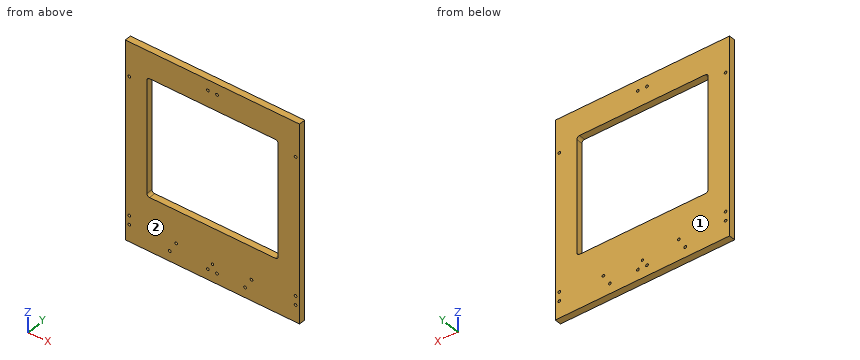
```python
from build123d import *

# Parameters (mm, degrees)
SKETCH_W        = 324
SKETCH_H        = 370
PAD_DEPTH       = 12
POCKET_DEPTH    = 12.001
SKETCH002_R     = 2.5
POCKET001_DEPTH = 12.001
SKETCH003_R     = 2.5
SKETCH003_R_2   = 2.25
POCKET002_DEPTH = 12.001


with BuildPart() as part:
    # Sketch → Pad (new body)
    with BuildSketch(Plane.XZ):
        with Locations((0, 185)):
            Rectangle(SKETCH_W, SKETCH_H)
    extrude(amount=PAD_DEPTH)

    # Sketch001 → Pocket (cut, through all)
    with BuildSketch(Plane.XZ.offset(12)):
        with BuildLine():
            ThreePointArc((-116.999969, 320), (-120.535523, 318.535545), (-122, 315))
            Line((-122, 315), (-122, 105))
            ThreePointArc((-122, 105), (-120.535523, 101.464455), (-116.999969, 100))
            Line((-116.999969, 100), (116.999969, 100))
            ThreePointArc((116.999969, 100), (120.535503, 101.464466), (121.999969, 105))
            Line((121.999969, 105), (121.999969, 315))
            ThreePointArc((121.999969, 315), (120.535503, 318.535534), (116.999969, 320))
            Line((-116.999969, 320), (116.999969, 320))
        make_face()
    extrude(amount=-POCKET_DEPTH, mode=Mode.SUBTRACT)

    # Sketch002 → Pocket001 (cut, through all)
    with BuildSketch(Plane.XZ.offset(12)):
        with Locations((-8.475, 19.5)):
            Circle(SKETCH002_R)
        with Locations((8.475, 19.5)):
            Circle(SKETCH002_R)
        with Locations((-8.475, 350.5)):
            Circle(SKETCH002_R)
        with Locations((8.475, 350.5)):
            Circle(SKETCH002_R)
        with Locations((154.5, 31.525)):
            Circle(SKETCH002_R)
        with Locations((154.5, 306)):
            Circle(SKETCH002_R)
        with Locations((-154.5, 306)):
            Circle(SKETCH002_R)
        with Locations((-154.5, 31.525)):
            Circle(SKETCH002_R)
        with Locations((-154.5, 48.475)):
            Circle(SKETCH002_R)
        with Locations((154.5, 48.475)):
            Circle(SKETCH002_R)
    extrude(amount=-POCKET001_DEPTH, mode=Mode.SUBTRACT)

    # Sketch003 → Pocket002 (cut, through all)
    with BuildSketch(Plane.XZ.offset(12)):
        with Locations((-79.45, 19)):
            Circle(SKETCH003_R)
        with Locations((-67.45, 39)):
            Circle(SKETCH003_R)
        with Locations((60.55, 19)):
            Circle(SKETCH003_R)
        with Locations((72.55, 39)):
            Circle(SKETCH003_R)
        with Locations((0, 32.85)):
            Circle(SKETCH003_R_2)
    extrude(amount=-POCKET002_DEPTH, mode=Mode.SUBTRACT)


solid = part.part
```
Verification items for the finished model (mm, model axes). Face numbers are marked on the shaded views. Give positions to 0.01 mm unless a question says otherwise; leave off trailing zeros. Loops run counter-clockwise (first coordinate to the right, second up) from the corner with the lowest first, then second, coordinate; pieces in that order, holes last. Notation, with made-up numbers: M 50.25,7.25 L 95.25,7.25 A27 ccw 95.25,45.25 Z; hole C -13.5,-25.5 d11. An arc over 180 degrees is marked long. One line per question, with ' | ' between items.
Item 1: Depth check by flat-ended pin: P1, Ø3, axis at x = 72.55, z = 39, coming from the +Y side. Enter the tip coordinate at first touch or a pass-through.
Completed:
P1: passes through
Item 2: Draft check along Y on the marked faces 1 and 2. Enter one of: +Y half, -Y half, draft (parallel to the pull), parting line (faces both ways), or undercut.
Completed:
face 1: +Y half | face 2: -Y half
Item 3: Section check C-C, the plane y = -10. State how many separate pieces and enclosed holes the cut face has, plus the area to 3 significant figures.
Completed:
separate pieces: 1 | enclosed holes: 16 | area: 65,900 mm^2
Item 4: Section check A-A, the plane x = -55. Record the cut outline in (y, z), plus the area to 3 significant figures.
Completed:
outline: M -12,0 L 0,0 L 0,100 L -12,100 Z; M -12,320 L 0,320 L 0,370 L -12,370 Z | area: 1,800 mm^2
Item 5: Section check B-B, the plane z = 128.5. Record the cut outline in (x, y).
Completed:
outline: M -162,-12 L -122,-12 L -122,0 L -162,0 Z; M 122,-12 L 162,-12 L 162,0 L 122,0 Z
Item 6: Thickness scan on line 1 (Z direction, x = -154.5, y = -6.5) (3 decimals); line 2 (X direction, y = -6, z = 306); line 3 (X direction, y = -2.25, z = 216.5). Record the ranges inside material, lowest first. Write a range as [from, to].
Completed:
line 1: z = [0, 29.025], [34.025, 45.975], [50.975, 303.5], [308.5, 370] | line 2: x = [-162, -157], [-152, -122], [122, 152], [157, 162] | line 3: x = [-162, -122], [122, 162]
